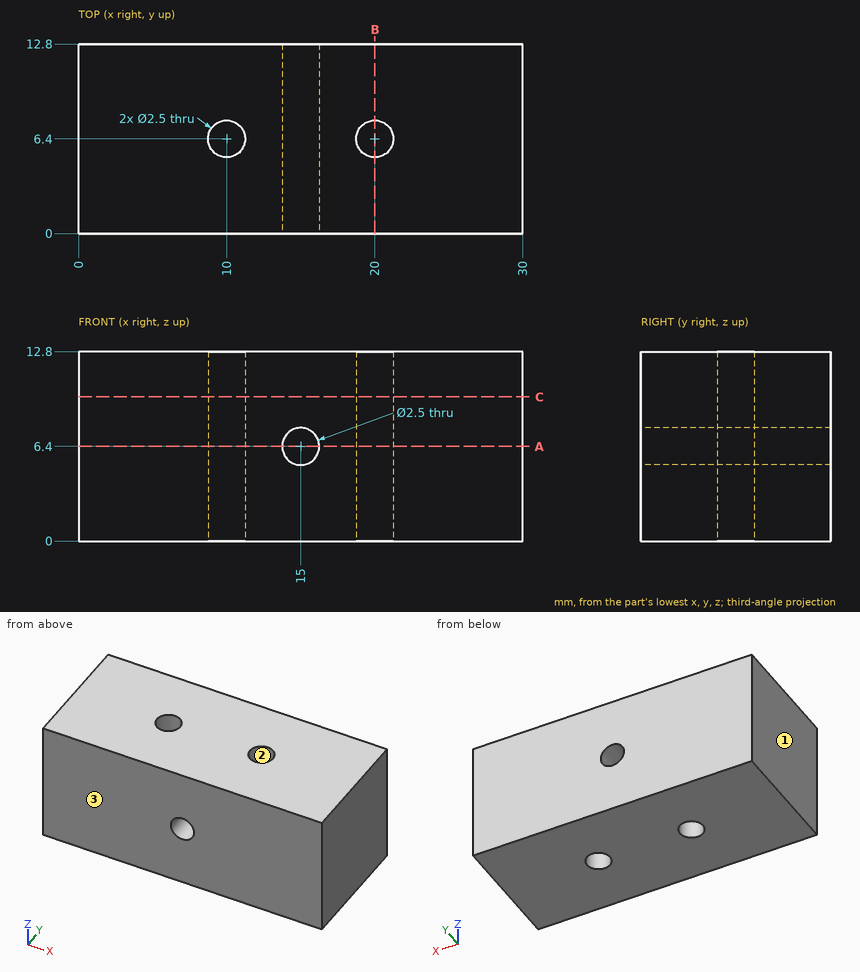
The drawing under review shows one solid part. Ordinate dimensions are in mm from its lowest x, y, z. Round coordinates to 2 decimals unless told otherwise and drop trailing zeros. Write each loop counter-clockwise with the first axis right and the second up, starting at its lowest first coordinate (ties: lowest second). Pieces come first, ordered by that corner, then holes. Notation, with made-up numbers: (-26, 4.25) - (27, 4.25) arc R25 cw to (27, 21.25) - close; hole circle Ø8 at (-37, -32.5). An arc over 180 degrees is marked (long way). Put each result on its own line as item: value.
Q1. We need section A-A (z = 6.4). Give the boundary of the cut face in (x, y).
Solved:
outline: (0, 0) - (13.75, 0) - (13.75, 12.8) - (0, 12.8) - close; (16.25, 0) - (30, 0) - (30, 12.8) - (16.25, 12.8) - close; hole circle Ø2.5 at (10, 6.4); hole circle Ø2.5 at (20, 6.4)
Q2. We need section C-C (z = 9.75). Give the boundary of the cut face in (x, y), and give its area (3 significant figures).
Solved:
outline: (0, 0) - (30, 0) - (30, 12.8) - (0, 12.8) - close; hole circle Ø2.5 at (10, 6.4); hole circle Ø2.5 at (20, 6.4)
area: 374 mm2
Q3. Insertion check: pin 1 Ø1.5 at (x, z) = (15, 6.4) entering from +Y. The pin has a flat end and moves straight along its axis. Give the tip position at first contact, or say it passes through.
Solved:
pin 1: passes through
Q4. Mouldability with a two-part tool opening along X and no side actions: class the marked faces 1, 2 and 3 as released by +X, released by -X, zero draft, split by the parting line, or undercut.
Solved:
face 1: released by -X
face 2: undercut
face 3: zero draft
Q5. Wall thickness on probe 1 along X at (y, z) = (6.4, 9.25); probe 2 along Y at (x, z) = (10, 7.25); probe 3 along X at (y, z) = (4.25, 6.4): over which ranges is each line inside the solid? List them lowest first.
Solved:
probe 1: x = 0 to 8.75, 11.25 to 18.75, 21.25 to 30
probe 2: y = 0 to 5.15, 7.65 to 12.8
probe 3: x = 0 to 13.75, 16.25 to 30
Q6. We need section B-B (x = 20). Give the boundary of the cut face in (y, z), and give its area (3 significant figures).
Solved:
outline: (0, 0) - (5.15, 0) - (5.15, 12.8) - (0, 12.8) - close; (7.65, 0) - (12.8, 0) - (12.8, 12.8) - (7.65, 12.8) - close
area: 132 mm2
